Model file for the job. Use its own axes, mm. Coordinates: 2 decimals unless noted, no trailing zeros. Write each loop counter-clockwise with the first axis right and the second up, starting at its lowest first coordinate (ties: lowest second). Pieces come first, ordered by that corner, then holes. Notation, with made-up numbers: (14.25, 45) -> (44.25, 45) arc R12 cw to (44.25, 67) -> close; hole circle Ø9 at (-3, 77.25). An arc over 180 degrees is marked (long way). Write item = value, one per line. Start each with the question number.
Autodesk Inventor part; units mm, degrees
ref_plane "YZ Plane" through (0, 0, 0) normal (1, 0, 0) x (0, 1, 0)
ref_plane "XZ Plane" through (0, 0, 0) normal (0, 1, 0) x (-1, 0, 0)
ref_plane "XY Plane" through (0, 0, 0) normal (0, 0, 1) x (1, 0, 0)
sketch "Absorber-Base" plane through (0, 0, 0) normal (0, 0, 1) x (1, 0, 0)
  line L0 (-9.2424, 9.2424) -> (9.2424, 9.2424)
  line L1 (9.2424, 9.2424) -> (9.2424, -9.2424)
  line L2 (9.2424, -9.2424) -> (-9.2424, -9.2424)
  line L3 (-9.2424, -9.2424) -> (-9.2424, 9.2424)
  line L4 (-9.2424, 9.2424) -> (9.2424, -9.2424) construction
  line L5 (9.2424, 9.2424) -> (-9.2424, -9.2424) construction
  point P0 (0, 0)
  dimension "d0" = 18.4849
extrude "Gesamtvolumen" add sketch "Absorber-Base" along normal blind 55
sketch "Skizze2" plane through (0, 0, 0) normal (0, 1, 0) x (-1, 0, 0)
  line L0 (-28, 0) -> (28, 0)
  line L1 (9.2424, 0) -> (9.2424, 55)
  line L2 (-9.2424, 0) -> (-9.2424, 55)
  line L3 (9.2424, 0) -> (-9.2424, 0)
  line L4 (-9.2424, 0) -> (-9.2424, 10)
  line L5 (-9.2424, 10) -> (9.2424, 10)
  line L6 (9.2424, 10) -> (9.2424, 0)
  line L7 (-9.2424, 55) -> (9.2424, 55)
  line L8 (0, 55) -> (9.2424, 10)
  line L9 (0, 55) -> (-9.2424, 10)
  point P0 (0, 0)
  point P1 (9.2424, 10)
  dimension "d6" = 10
extrude "Cutaway" cut sketch "Skizze2" along normal mid plane 18.4848 contours L2 L7 L9 | L8 L7 L1
pattern_circular "Runde Anordnung1" count 2 over 90 about axis through (0, 0, -10) along (0, 0, 1) of "Cutaway"
equation "\"d0\" = Base_Seitenlänge"
equation "\"d1\" = Gesamthöhe"
equation "\"d6\" = Base_Höhe"
equation "\"d7\" = Base_Seitenlänge"
equation "\"Base_Seitenlänge\" = 18.48485"
equation "\"Base_Höhe\" = 10"
equation "\"Gesamthöhe\" = 55"
properties part number "Absorber - SEA-PM5"
(1) Saw through at D-D (z = 10.5). Give the cut face in (x, y), then the cut area to 3 significant figures.
(2) Saw through at A-A (y = 0.5). Give the cut face in (x, z).
(3) Saw through at B-B (x = 1.75). Give the cut face in (y, z).
(4) Saw through at C-C (z = 51). Give the cut face in (x, y), then the cut area to 3 significant figures.
(5) Drill centre lines: line 1 along X through (y, z) = (-6.5, 10.5); line 2 along Y through (x, z) = (3, 13.5); line 3 along X through (y, z) = (0, 33.5). Where is each one in solid material? Low to high.
(6) Drop flat-ended pins along their axis: pin 1 Ø1.5 at (x, z) = (-5.5, 19.5) entering from -Y; pin 2 Ø4 at (y, z) = (3, 49) entering from +X; pin 3 Ø1.5 at (x, z) = (1, 43) entering from +Y. Give the stop position or say it passes through.
Returned:
q1.outline = (-9.14, -9.14) -> (9.14, -9.14) -> (9.14, 9.14) -> (-9.14, 9.14) -> close
q1.area = 334 mm2
q2.outline = (-9.24, 0) -> (9.24, 0) -> (9.24, 10) -> (0.5, 52.57) -> (-0.5, 52.57) -> (-9.24, 10) -> close
q3.outline = (-9.24, 0) -> (9.24, 0) -> (9.24, 10) -> (1.75, 46.48) -> (-1.75, 46.48) -> (-9.24, 10) -> close
q4.outline = (-0.82, -0.82) -> (0.82, -0.82) -> (0.82, 0.82) -> (-0.82, 0.82) -> close
q4.area = 2.70 mm2
q5.line_1 = -9.14 to 9.14
q5.line_2 = -8.52 to 8.52
q5.line_3 = -4.42 to 4.42
q6.pin_1 = -7.45
q6.pin_2 = 1.51
q6.pin_3 = 2.62
